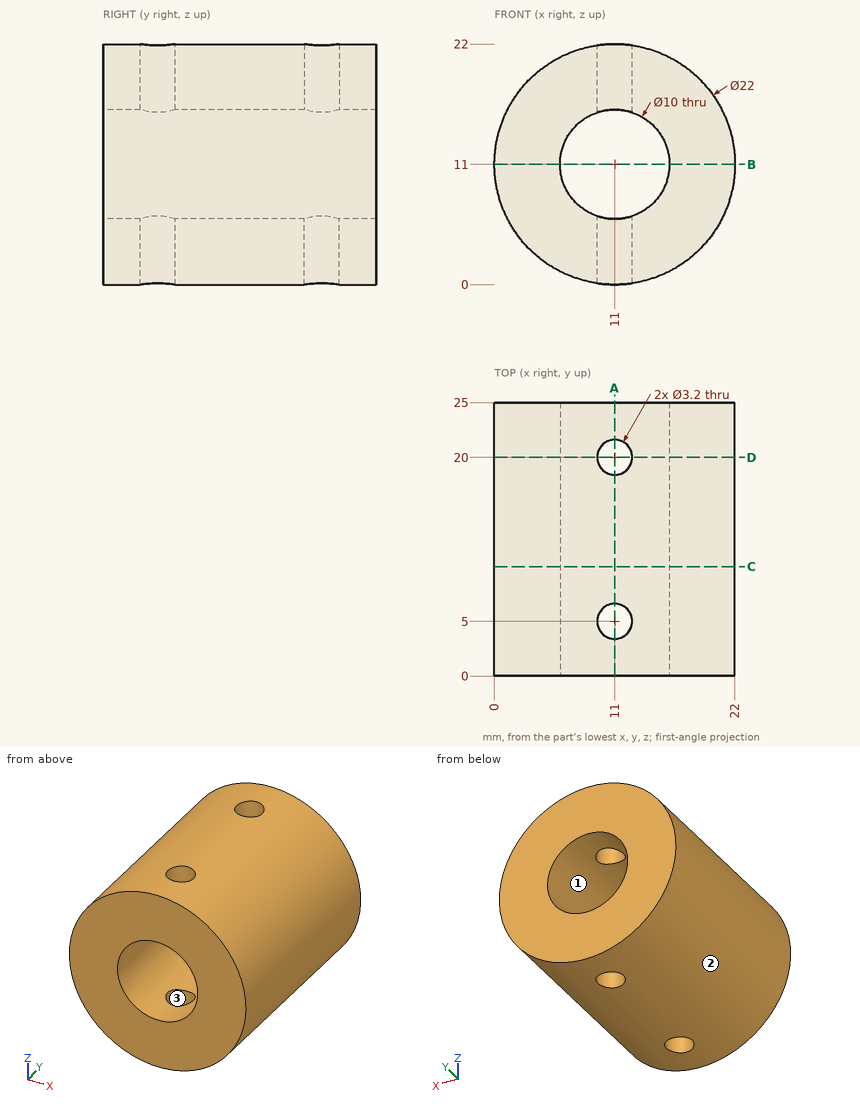
For this review, use the dimensioned drawing (mm, ordinates from the lowest corner) and the shaded views. Coordinates: 2 decimals unless noted, no trailing zeros. Write each loop counter-clockwise with the first axis right and the second up, starting at its lowest first coordinate (ties: lowest second). Pieces come first, ordered by that corner, then holes. Notation, with made-up numbers: (67.25, 63.5) - (101.25, 63.5) arc R14 cw to (101.25, 77.5) - close; hole circle Ø3 at (54, 68.25). An arc over 180 degrees is marked (long way). Answer as a JSON object with one key per item and string values. Group by question number.
1. Clearance check with flat-ended pins moving along their axes: pin 1 Ø2 at (y, z) = (8, 9) entering from +X; pin 2 Ø1.9 at (x, y) = (11, 5) entering from +Z; pin 3 Ø1 at (y, z) = (16, 14.5) entering from -X; pin 4 Ø1.5 at (x, y) = (3.5, 15) entering from -Z. State where each tip first meets the part, or that it passes through.
2. To check wall thickness, follow probe 1 along X at (y, z) = (7.5, 11); probe 2 along Z at (x, y) = (9, 12.25); probe 3 along Z at (x, y) = (9.75, 23.5). State the ranges of each line that lie inside material, in increasing order.
3. Add section C-C (y = 10). Give the boundary of the cut face in (x, z).
4. Mouldability with a two-part tool opening along Z and no side actions: class the marked faces 1, 2 and 3 as pulls with the +Z half, pulls with the -Z half, needs draft (parallel to the pull), parting line crosses it, or undercut.
5. Add section B-B (z = 11). Give the boundary of the cut face in (x, y), plus the area to 3 significant figures.
6. Add section A-A (x = 11). Give the boundary of the cut face in (y, z).
7. Add section D-D (y = 20). Give the boundary of the cut face in (x, z).
Findings:
{
 "1": {"pin 1": "x = 21.95", "pin 2": "through", "pin 3": "x = 0.42", "pin 4": "z = 2.31"},
 "2": {"probe 1": "0 to 6, 16 to 22", "probe 2": "0.18 to 6.42, 15.58 to 21.82", "probe 3": "0.07 to 6.16, 15.84 to 21.93"},
 "3": {"outline": "circle Ø22 at (11, 11); hole circle Ø10 at (11, 11)"},
 "4": {"face 1": "undercut", "face 2": "parting line crosses it", "face 3": "needs draft"},
 "5": {"outline": "(0, 0) - (6, 0) - (6, 25) - (0, 25) - close; (16, 0) - (22, 0) - (22, 25) - (16, 25) - close", "area": "300 mm²"},
 "6": {"outline": "(0, 0) - (3.4, 0) - (3.4, 6) - (0, 6) - close; (0, 16) - (3.4, 16) - (3.4, 22) - (0, 22) - close; (6.6, 0) - (18.4, 0) - (18.4, 6) - (6.6, 6) - close; (6.6, 16) - (18.4, 16) - (18.4, 22) - (6.6, 22) - close; (21.6, 0) - (25, 0) - (25, 6) - (21.6, 6) - close; (21.6, 16) - (25, 16) - (25, 22) - (21.6, 22) - close"},
 "7": {"outline": "(9.4, 0.12) - (9.4, 6.26) arc R5 cw to (9.4, 15.74) - (9.4, 21.88) arc R11 ccw to start; (12.6, 0.12) arc R11 ccw to (12.6, 21.88) - (12.6, 15.74) arc R5 cw to (12.6, 6.26) - close"}
}
